Could you check a few things on this model? Use its own coordinates, in mm. A direction names the side the tool comes from. Coordinates: 2 decimals unless noted, no trailing zeros. Order: outer loops, then holes, each group sorted by start corner. A loop starts at its lowest first (then second) coordinate and runs counter-clockwise, first axis right, second up. Notation, with made-up numbers: (80.25, -32.75) -> (126.25, -32.75) arc R27 cw to (126.25, -5.75) -> close; hole circle Ø3 at (-29.5, 25). An arc over 180 degrees is marked (long way). Use a Markdown table: item, result. Add a question column.
1) If we section it at D-D (z = 43): Write out the boundary of the cut face in (x, y), plus the area to 3 significant figures.
2) Thinking about a two-plate mould opening in Y: for faces 4 (the cylindrical face through (1.48, 180.72, 81.54)), 5 (the flat face through (0, 94, 49)), 6 (the cylindrical face through (1.521, 39.974, 119.941)), which applies, +Y half, -Y half, draft (parallel to the pull), parting line (faces both ways), or undercut?
3) If we section it at B-B (z = 104): Write out the boundary of the cut face in (x, y), plus the area to 3 significant figures.
4) If we section it at C-C (y = 182.77): Write out the boundary of the cut face in (x, z).
5) If I drill on L1, parallel to Z at x = 2, y = 162.91; L2, parallel to Y at x = 1.85, z = 124.55; L3, parallel to Y at x = 2, z = 119.55, over which ranges is the centre line in solid material (lowest first)? Write a range as [from, to].
6) Will these pins go through, and if not, where does the flat tip stop? pin 1 Ø2.5 at (x, z) = (-6.5, 71.5) entering from -Y; pin 2 Ø3.5 at (y, z) = (162.91, 119.55) entering from +X; pin 3 Ø5.5 at (y, z) = (182.77, 82) entering from -X; pin 4 Ø1.6 at (x, y) = (2, 54.5) entering from +Z.
7) If we section it at A-A (y = 89.5): Write out the boundary of the cut face in (x, z), plus the area to 3 significant figures.
8) Which directions (+Z, -Z, +X, -X, +Y, -Y) give clear straight access to the entire face, cutting with the end or side of a thin tool? Please do faces 1 (the flat face through (-7, 135, 72)), 2 (the flat face through (3, 94, 49)), 3 (the flat face through (-5, 94, 70)).
```python
from build123d import *

# Parameters (mm, degrees)
SKETCH_2_W               = 3
SKETCH_2_H               = 190
SM_BASE_FLANGE_1_DEPTH   = 89.2
SKETCH_14_W              = 16.2
SKETCH_14_H              = 80
CUT_EXTRUDE_2_DEPTH      = 10
SM_START                 = 53.5
SM_EDGE_FLANGE_1_DEPTH   = 83
SM_EDGE_FLANGE_1_2_DEPTH = 1.5
SM_START_2               = 135
SM_EDGE_FLANGE_1_3_DEPTH = 1.5
SM_START_3               = 55
SM_EDGE_FLANGE_1_4_DEPTH = 80
CUT_EXTRUDE_START        = -1.5
SKETCH_18_W              = 3
SKETCH_18_H              = 16.2
CUT_EXTRUDE_3_DEPTH      = 1.5
SKETCH_19_W              = 3
SKETCH_19_H              = 16.2
CUT_EXTRUDE_4_DEPTH      = 1.5
CUT_EXTRUDE_5_DEPTH      = 10
HOLE_WIZARD_M4_2_D       = 3.3
HOLE_WIZARD_M4_2_DEPTH   = 10.1
HOLE_WIZARD_M4_2_TIP     = 0.991420021
HOLE_WIZARD_M5_1_D       = 4.2
HOLE_WIZARD_M5_1_DEPTH   = 12.4
HOLE_WIZARD_M5_1_TIP     = 1.2618073
SKETCH_25_W              = 3
SKETCH_25_H              = 53.5
EXTRUDE_1_DEPTH          = 40
SKETCH_26_R              = 3
CUT_EXTRUDE_6_DEPTH      = 3
PATTERN_LINEAR_1_COUNT   = 2
PATTERN_LINEAR_1_PITCH   = 15.55
SKETCH_27_R              = 3
CUT_EXTRUDE_7_DEPTH      = 231.635296518
HOLE_WIZARD_M4_3_D       = 3.3
HOLE_WIZARD_M4_3_DEPTH   = 10.1
HOLE_WIZARD_M4_3_TIP     = 0.991420021


# Read off the part's stored shape, not the designer's step: 边线-法兰1
# Sheet-metal steps are written as plain solids
with BuildPart() as part:
    # Sketch 2 → 基体-法兰1 (new body)
    with BuildSketch(Plane.XY):
        with Locations((1.5, 95)):
            Rectangle(SKETCH_2_W, SKETCH_2_H)
    extrude(amount=SM_BASE_FLANGE_1_DEPTH)

    # 草图14 → 切除-拉伸2 (cut)
    with BuildSketch(Plane(origin=(3, 0, 0), x_dir=(0, 0, -1), z_dir=(1, 0, 0))):
        with Locations((-81.1, 95)):
            Rectangle(SKETCH_14_W, SKETCH_14_H)
    extrude(amount=-CUT_EXTRUDE_2_DEPTH, mode=Mode.SUBTRACT)

    # 边线-法兰1 outline → 边线-法兰1 (cut)
    with BuildSketch(Plane(origin=(0, 0, 0), x_dir=(1, 0, 0), z_dir=(0, 1, 0)).offset(SM_START)):
        with BuildLine():
            Line((3, -73), (3, -69.2634))
            ThreePointArc((3, -69.2634), (2.154295979, -71.630867001), (0, -72.926677222))
            Line((0, -72.926677222), (0, -73))
            Line((0, -73), (3, -73))
        make_face()
    extrude(amount=SM_EDGE_FLANGE_1_DEPTH, mode=Mode.SUBTRACT)

    # Sm Edge Flange 1 2 outline → Sm Edge Flange 1 2 (cut)
    with BuildSketch(Plane(origin=(0, 0, 0), x_dir=(1, 0, 0), z_dir=(0, 1, 0)).offset(SM_START)):
        with BuildLine():
            Line((3, -67.7634), (0, -67.7634))
            Line((0, -67.7634), (0, -72.926677222))
            ThreePointArc((0, -72.926677222), (2.154295979, -71.630867001), (3, -69.2634))
            Line((3, -69.2634), (3, -67.7634))
        make_face()
    extrude(amount=SM_EDGE_FLANGE_1_2_DEPTH, mode=Mode.SUBTRACT)

    # Sm Edge Flange 1 3 outline → Sm Edge Flange 1 3 (cut)
    with BuildSketch(Plane(origin=(0, 0, 0), x_dir=(1, 0, 0), z_dir=(0, 1, 0)).offset(SM_START_2)):
        with BuildLine():
            Line((3, -67.7634), (0, -67.7634))
            Line((0, -67.7634), (0, -72.926677222))
            ThreePointArc((0, -72.926677222), (2.154295979, -71.630867001), (3, -69.2634))
            Line((3, -69.2634), (3, -67.7634))
        make_face()
    extrude(amount=SM_EDGE_FLANGE_1_3_DEPTH, mode=Mode.SUBTRACT)

    # Sm Edge Flange 1 4 outline → Sm Edge Flange 1 4 (add)
    with BuildSketch(Plane(origin=(0, 0, 0), x_dir=(1, 0, 0), z_dir=(0, 1, 0)).offset(SM_START_3)):
        with BuildLine():
            Line((0, -72.926677222), (0, -69.2634))
            ThreePointArc((0, -69.2634), (-0.215745145, -69.784254855), (-0.7366, -70))
            Line((-0.7366, -70), (-17, -70))
            Line((-17, -70), (-17, -73))
            Line((-17, -73), (-0.7366, -73))
            ThreePointArc((-0.7366, -73), (-0.36647982, -72.981624121), (0, -72.926677222))
        make_face()
    extrude(amount=SM_EDGE_FLANGE_1_4_DEPTH)

    # 草图18 → 切除-拉伸3 (cut)
    with BuildSketch(Plane.XZ.offset(-135).offset(CUT_EXTRUDE_START)):
        with Locations((1.5, 81.1)):
            Rectangle(SKETCH_18_W, SKETCH_18_H)
    extrude(amount=CUT_EXTRUDE_3_DEPTH, mode=Mode.SUBTRACT)

    # 草图19 → 切除-拉伸4 (cut)
    with BuildSketch(Plane(origin=(0, 55, 0), x_dir=(1, 0, 0), z_dir=(0, 1, 0)).offset(CUT_EXTRUDE_START)):
        with Locations((1.5, -81.1)):
            Rectangle(SKETCH_19_W, SKETCH_19_H)
    extrude(amount=CUT_EXTRUDE_4_DEPTH, mode=Mode.SUBTRACT)

    # 草图20 → 切除-拉伸5 (cut)
    with BuildSketch(Plane(origin=(0, 0, 70), x_dir=(-1, 0, 0), z_dir=(0, 0, -1))):
        with BuildLine():
            Line((6.25, 80), (6.25, 110))
            ThreePointArc((6.25, 110), (9, 112.75), (11.75, 110))
            Line((11.75, 110), (11.75, 80))
            ThreePointArc((11.75, 80), (9, 77.25), (6.25, 80))
        make_face()
    extrude(amount=-CUT_EXTRUDE_5_DEPTH, mode=Mode.SUBTRACT)

    # M4 螺纹孔2
    with Locations(Plane(origin=(3, 0, 0), x_dir=(0, 0, -1), z_dir=(1, 0, 0))):
        with Locations((-31.544019194, 25), (-16.544019194, 25), (-31.544019194, 55), (-16.544019194, 55), (-16.544019194, 135), (-31.544019194, 135), (-16.544019194, 165), (-31.544019194, 165)):
            Hole(HOLE_WIZARD_M4_2_D / 2, depth=HOLE_WIZARD_M4_2_DEPTH)
            with Locations((0, 0, -(HOLE_WIZARD_M4_2_DEPTH + HOLE_WIZARD_M4_2_TIP / 2))):  # 118° drill point
                Cone(0, HOLE_WIZARD_M4_2_D / 2, HOLE_WIZARD_M4_2_TIP, mode=Mode.SUBTRACT)

    # M5 螺纹孔1
    with Locations(Plane(origin=(3, 0, 0), x_dir=(0, 0, -1), z_dir=(1, 0, 0))):
        with Locations((-82, 170.77), (-82, 182.77)):
            Hole(HOLE_WIZARD_M5_1_D / 2, depth=HOLE_WIZARD_M5_1_DEPTH)
            with Locations((0, 0, -(HOLE_WIZARD_M5_1_DEPTH + HOLE_WIZARD_M5_1_TIP / 2))):  # 118° drill point
                Cone(0, HOLE_WIZARD_M5_1_D / 2, HOLE_WIZARD_M5_1_TIP, mode=Mode.SUBTRACT)

    # 草图25 → 凸台-拉伸1 (add)
    with BuildSketch(Plane.XY.offset(89.2)):
        with Locations((1.5, 163.25)):
            Rectangle(SKETCH_25_W, SKETCH_25_H)
        with Locations((1.5, 26.75)):
            Rectangle(SKETCH_25_W, SKETCH_25_H)
    extrude(amount=EXTRUDE_1_DEPTH)

    # 草图26 → 切除-拉伸6 (cut)
    with BuildSketch(Plane(origin=(3, 0, 0), x_dir=(0, 0, -1), z_dir=(1, 0, 0))):
        with Locations((-119.55, 162.91)):
            Circle(SKETCH_26_R)
    cut_extrude_6 = extrude(amount=-CUT_EXTRUDE_6_DEPTH, mode=Mode.SUBTRACT)

    # 阵列(线性)1: 切除-拉伸6 ×2
    with Locations(*[(0, 0, -i * PATTERN_LINEAR_1_PITCH) for i in range(1, PATTERN_LINEAR_1_COUNT)]):
        add(cut_extrude_6, mode=Mode.SUBTRACT)

    # 草图27 → 切除-拉伸7 (cut, through all)
    with BuildSketch(Plane(origin=(3, 0, 0), x_dir=(0, 0, -1), z_dir=(1, 0, 0))):
        with Locations((-104, 37)):
            Circle(SKETCH_27_R)
        with Locations((-119.55, 37)):
            Circle(SKETCH_27_R)
    extrude(amount=-CUT_EXTRUDE_7_DEPTH, mode=Mode.SUBTRACT)

    # M4 螺纹孔3
    with Locations(Plane(origin=(3, 0, 0), x_dir=(0, 0, -1), z_dir=(1, 0, 0))):
        with Locations((-124.55, 16.7), (-124.55, 7.7)):
            Hole(HOLE_WIZARD_M4_3_D / 2, depth=HOLE_WIZARD_M4_3_DEPTH)
            with Locations((0, 0, -(HOLE_WIZARD_M4_3_DEPTH + HOLE_WIZARD_M4_3_TIP / 2))):  # 118° drill point
                Cone(0, HOLE_WIZARD_M4_3_D / 2, HOLE_WIZARD_M4_3_TIP, mode=Mode.SUBTRACT)


solid = part.part
```
Answer sheet:
| question | item | result |
|---|---|---|
| 1 | outline | (0, 0) -> (3, 0) -> (3, 190) -> (0, 190) -> close |
| 1 | area | 570 mm2 |
| 2 | face 4 | undercut |
| 2 | face 5 | draft |
| 2 | face 6 | undercut |
| 3 | outline | (0, 0) -> (3, 0) -> (3, 34) -> (0, 34) -> close; (0, 40) -> (3, 40) -> (3, 53.5) -> (0, 53.5) -> close; (0, 136.5) -> (3, 136.5) -> (3, 159.91) -> (0, 159.91) -> close; (0, 165.91) -> (3, 165.91) -> (3, 190) -> (0, 190) -> close |
| 3 | area | 285 mm2 |
| 4 | outline | (0, 0) -> (3, 0) -> (3, 79.9) -> (0, 79.9) -> close; (0, 84.1) -> (3, 84.1) -> (3, 129.2) -> (0, 129.2) -> close |
| 5 | L1 | [0, 101], [107, 116.55], [122.55, 129.2] |
| 5 | L2 | [0, 6.05], [9.35, 15.05], [18.35, 53.5], [136.5, 190] |
| 5 | L3 | [0, 34], [40, 53.5], [136.5, 159.91], [165.91, 190] |
| 6 | pin 1 | y = 55 |
| 6 | pin 2 | through |
| 6 | pin 3 | x = 0 |
| 6 | pin 4 | z = 72.35 |
| 7 | outline | (-17, 70) -> (-11.75, 70) -> (-11.75, 73) -> (-17, 73) -> close; (-6.25, 70) -> (-0.74, 70) arc R0.74 cw to (0, 69.26) -> (0, 0) -> (3, 0) -> (3, 69.26) arc R3.74 ccw to (-0.74, 73) -> (-6.25, 73) -> close |
| 7 | area | 251 mm2 |
| 8 | face 1 | +Z, +X, -X |
| 8 | face 2 | +Z, -Z, +X, +Y, -Y |
| 8 | face 3 | -Z, -X, +Y, -Y |
